Could you check a few things on this drawing? It's one solid part, dimensions in mm from its lowest x, y, z. Coordinates: 2 decimals unless noted, no trailing zeros. Write each loop counter-clockwise with the first axis right and the second up, starting at its lowest first coordinate (ties: lowest second). Pieces come first, ordered by that corner, then holes.
Item 1: I want a section at B-B (z = 14). Please give me the cut outline in (x, y), and give its area (3 significant figures).
Item 2: I want a section at C-C (y = 6.75). Count the separate pieces of the cut face and the enclosed holes in it, and give its area (3 significant figures).
Item 3: I want a section at D-D (z = 7.5). Please give me the cut outline in (x, y) (1 decimal), and give its area (3 significant figures).
Item 4: I'm going to push flat-ended pins straight in: P1, Ø1, axis at y = 16, z = 7, coming from the -X side (1 decimal); P2, Ø8, axis at y = 15, z = 3, coming from the +X side; P3, Ø3, axis at y = 15, z = 22, coming from the +X side. Where does each tip first touch, or does it pass through?
Item 5: I want a section at A-A (x = 15). Please give me the cut outline in (y, z).
Item 6: If we mould it in two halves opening along Z, with no side actions, what happens to the marked faces 1, 2 and 3? For each: pulls with the +Z half, pulls with the -Z half, needs draft (parallel to the pull), parting line crosses it, or undercut.
Item 7: Please list where these lines run through material, in increasing order: line 1 (X direction, y = 9, z = 19.75) (1 decimal); line 2 (X direction, y = 6.5, z = 20) (1 decimal); line 3 (Z direction, x = 34.5, y = 10) (1 decimal).
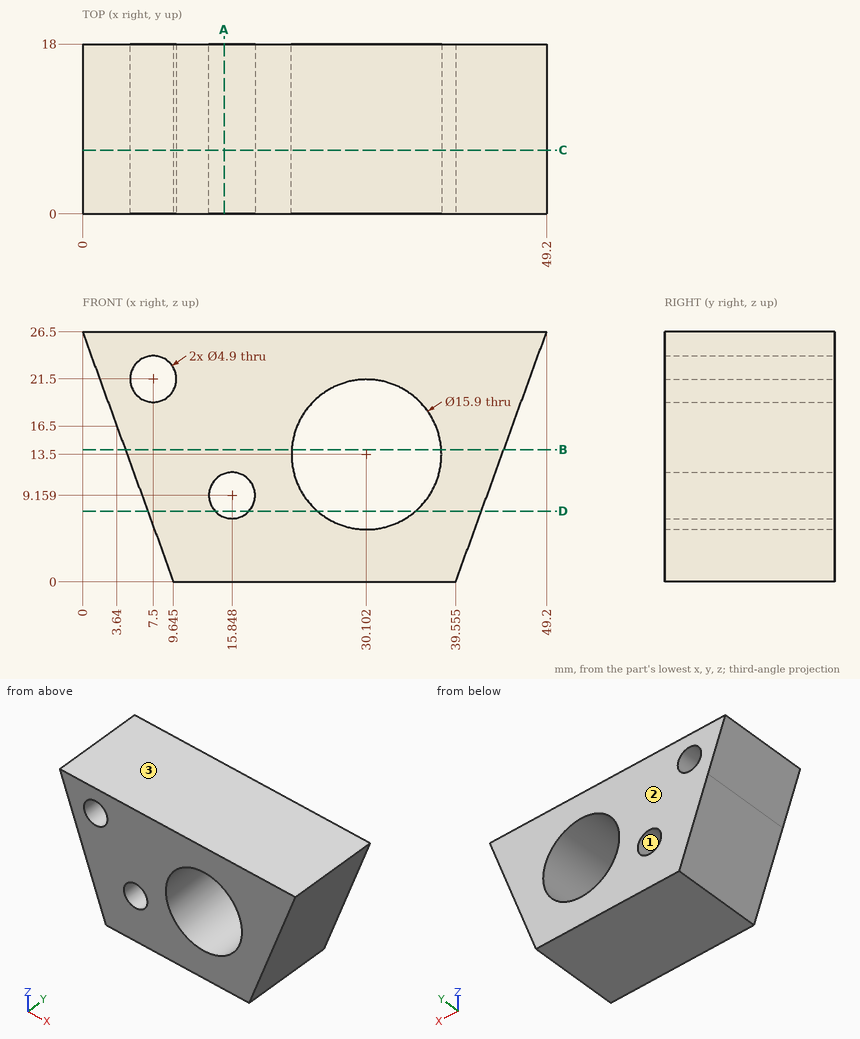
Answer:
1. outline: (4.55, 0) - (22.17, 0) - (22.17, 18) - (4.55, 18) - close; (38.04, 0) - (44.65, 0) - (44.65, 18) - (38.04, 18) - close
1. area: 436 mm2
2. separate pieces: 1
2. enclosed holes: 3
2. area: 812 mm2
3. outline: (6.9, 0) - (14, 0) - (14, 18) - (6.9, 18) - close; (17.7, 0) - (24.9, 0) - (24.9, 18) - (17.7, 18) - close; (35.3, 0) - (42.3, 0) - (42.3, 18) - (35.3, 18) - close
3. area: 384 mm2
4. P1: stops at x = 6.9
4. P2: stops at x = 42.1
4. P3: stops at x = 48.11
5. outline: (0, 0) - (18, 0) - (18, 6.86) - (0, 6.86) - close; (0, 11.46) - (18, 11.46) - (18, 26.5) - (0, 26.5) - close
6. face 1: undercut
6. face 2: needs draft
6. face 3: pulls with the +Z half
7. line 1: x = 2.5 to 5.8, 9.2 to 25.2, 35 to 46.7
7. line 2: x = 2.4 to 5.6, 9.4 to 25.5, 34.7 to 46.8
7. line 3: z = 0 to 6.9, 20.1 to 26.5
